from build123d import *

# Parameters (mm, degrees)
BOSS_EXTRUDE1_DEPTH = 279.4


with BuildPart() as part:
    # Sketch1 → Boss-Extrude1 (new body)
    with BuildSketch(Plane.XY):
        with BuildLine():
            Line((46.99, -39.37), (47.78375, -39.37))
            Line((47.78375, -39.37), (47.78375, -40.16375))
            ThreePointArc((47.78375, -40.16375), (45.551903673, -45.551903673), (40.16375, -47.78375))
            Line((40.16375, -47.78375), (-40.16375, -47.78375))
            ThreePointArc((-40.16375, -47.78375), (-45.551903673, -45.551903673), (-47.78375, -40.16375))
            Line((-47.78375, -40.16375), (-47.78375, -39.37))
            Line((-47.78375, -39.37), (-46.99, -39.37))
            ThreePointArc((-46.99, -39.37), (-44.758153673, -44.758153673), (-39.37, -46.99))
            Line((-39.37, -46.99), (39.37, -46.99))
            ThreePointArc((39.37, -46.99), (44.758153673, -44.758153673), (46.99, -39.37))
        make_face()
    extrude(amount=BOSS_EXTRUDE1_DEPTH)


solid = part.part
Verification items for the finished model (mm, model axes). A direction names the side the tool comes from. Give positions to 0.01 mm unless a question says otherwise; leave off trailing zeros. Write each loop counter-clockwise with the first axis right and the second up, starting at its lowest first coordinate (ties: lowest second). Pieces come first, ordered by that corner, then holes. Notation, with made-up numbers: M -8.75,8 L 1.25,8 A17 cw 1.25,37 Z; hole C -14.5,39 d7. An arc over 180 degrees is marked long. Use CSV: the item, a comma, the result in double quotes.
1) Material ranges on line 1 along X through (y, z) = (-40, 213.5); line 2 along Y through (x, z) = (3, 100.5); line 3 along X through (y, z) = (-43.75, 229.5), recorded low to high.
Final values:
line 1,"-47.78 to -46.96, 46.96 to 47.78"
line 2,"-47.78 to -46.99"
line 3,"-46.89 to -45.61, 45.61 to 46.89"
2) Cross-section at A-A (y = -43). Enter the section's corners in (x, z), plus the area to 3 significant figures.
Final values:
outline,"M -47.24,0 L -46.07,0 L -46.07,279.4 L -47.24,279.4 Z; M 46.07,0 L 47.24,0 L 47.24,279.4 L 46.07,279.4 Z"
area,"652 mm²"
3) Release check for a two-part mould opening along X. For faces 3 (the face through (45.611, -45.492, 137.744)), 4 (the face through (-45.492, -45.611, 137.744)), 5 (the face through (0.2, -47.3, 279.4)), 6 (the face through (-1, -46.99, 138)) record: released by +X, released by -X, zero draft, split by the parting line, or undercut.
Final values:
face 3,"released by +X"
face 4,"released by -X"
face 5,"zero draft"
face 6,"undercut"
4) Go/stop test with flat-tipped pins: pin 1 Ø1.5 at (y, z) = (-42.5, 175) entering from -X; pin 2 Ø5 at (y, z) = (-43, 232.5) entering from +X; pin 3 Ø1.5 at (y, z) = (-43.5, 76) entering from -X. Record where each tip stops, or that it passes through.
Final values:
pin 1,"x = -47.62"
pin 2,"x = 47.78"
pin 3,"x = -47.33"
5) Cross-section at C-C (x = -20.5). Enter the section's corners in (y, z).
Final values:
outline,"M -47.78,0 L -46.99,0 L -46.99,279.4 L -47.78,279.4 Z"
6) Access from +Z, -Z, +X, -X, +Y, -Y to the whole of each face (thin tool, end or side, straight path). Record for faces 1 (the face through (44.699, -44.817, 137.744)), 2 (the face through (1, -47.784, 138)).
Final values:
face 1,"+Z, -Z, +Y"
face 2,"+Z, -Z, +X, -X, -Y"
7) Cross-section at B-B (z = 225.5). Enter the section's corners in (x, y), plus the area to 3 significant figures.
Final values:
outline,"M -47.78,-40.16 A7.62 ccw -40.16,-47.78 L 40.16,-47.78 A7.62 ccw 47.78,-40.16 L 47.78,-39.37 L 46.99,-39.37 A7.62 cw 39.37,-46.99 L -39.37,-46.99 A7.62 cw -46.99,-39.37 L -47.78,-39.37 Z"
area,"88.0 mm²"
